Source: three-view drawing plus pictorial views. Frame: mm from the lowest corner of the part. A direction names the side the tool comes from. Coordinates: 2 decimals unless noted, no trailing zeros. Loops run counter-clockwise (first coordinate to the right, second up) from the corner with the lowest first, then second, coordinate; pieces in that order, holes last.
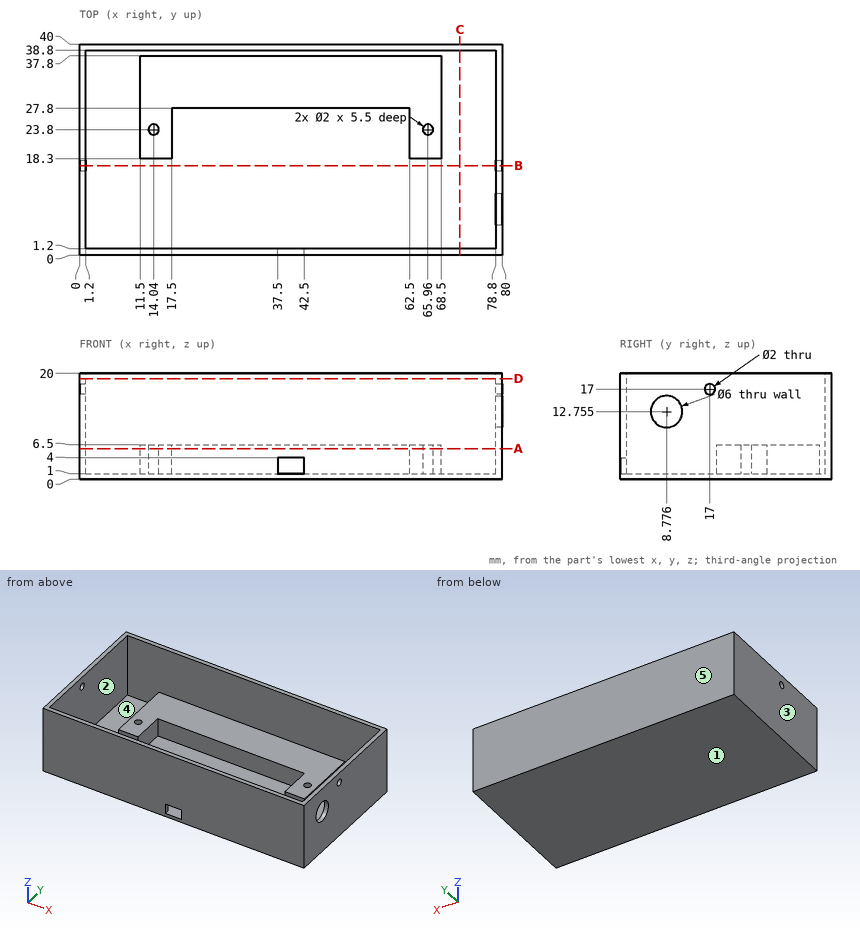
Q1. Section query D-D on z = 19. Return the cut outline in (x, y).
Q2. Reachability of the marked faces 1 and 2 from +Z, -Z, +X, -X, +Y, -Y: full face, straight path, thin tool, end or side. Return the list, or none.
Q3. Section query A-A on z = 5.75. Return the cut outline in (x, y).
Q4. Material intervals for line 1 along X through (y, z) = (20, 2.75); line 2 along Y through (x, z) = (14.04, 4.7); line 3 along Y through (x, z) = (13, 5.5), sorted ascending.
Q5. Draft query along Y for the marked faces 3, 4 and 5. Return one class per face: released by +Y, released by -Y, zero draft, split by the parting line, or undercut.
Q6. Section query C-C on x = 72. Return the cut outline in (y, z).
Q7. First-contact query: pin 1 Ø1 at (x, y) = (48, 7) entering from +Z; pin 2 Ø1.8 at (y, z) = (17, 17) entering from +X; pin 3 Ø5.5 at (y, z) = (8.78, 12.76) entering from +X. Flat tips, straight axial feed; report the tip coordinate or a pass-through.
Q8. Section query B-B on y = 17. Return the cut outline in (x, z).
Resolved:
1. outline: (0, 0) - (80, 0) - (80, 40) - (0, 40) - close; hole (1.2, 1.2) - (78.8, 1.2) - (78.8, 38.8) - (1.2, 38.8) - close
2. face 1: -Z, +X, -X, +Y, -Y
2. face 2: +Z
3. outline: (0, 0) - (80, 0) - (80, 40) - (0, 40) - close; (11.5, 18.3) - (17.5, 18.3) - (17.5, 27.8) - (62.5, 27.8) - (62.5, 18.3) - (68.5, 18.3) - (68.5, 37.8) - (11.5, 37.8) - close; hole (1.2, 1.2) - (78.8, 1.2) - (78.8, 38.8) - (1.2, 38.8) - close; hole circle Ø2 at (14.04, 23.8); hole circle Ø2 at (65.96, 23.8)
4. line 1: x = 0 to 1.2, 11.5 to 17.5, 62.5 to 68.5, 78.8 to 80
4. line 2: y = 0 to 1.2, 18.3 to 22.8, 24.8 to 37.8, 38.8 to 40
4. line 3: y = 0 to 1.2, 18.3 to 37.8, 38.8 to 40
5. face 3: zero draft
5. face 4: undercut
5. face 5: released by +Y
6. outline: (0, 0) - (40, 0) - (40, 20) - (38.8, 20) - (38.8, 1) - (1.2, 1) - (1.2, 20) - (0, 20) - close
7. pin 1: stops at z = 1
7. pin 2: passes through
7. pin 3: stops at x = 1.2
8. outline: (0, 0) - (80, 0) - (80, 16) - (78.8, 16) - (78.8, 1) - (1.2, 1) - (1.2, 16) - (0, 16) - close; (0, 18) - (1.2, 18) - (1.2, 20) - (0, 20) - close; (78.8, 18) - (80, 18) - (80, 20) - (78.8, 20) - close
